Model file for the job. Use its own axes, mm. A direction names the side the tool comes from. Give positions to 0.01 mm unless a question says otherwise; leave off trailing zeros. Loops run counter-clockwise (first coordinate to the right, second up) from the corner with the lowest first, then second, coordinate; pieces in that order, holes last. Notation, with made-up numbers: (68.25, 44.5) - (104.25, 44.5) arc R27 cw to (104.25, 73.5) - close; hole circle Ø1 at (82, 22). An arc over 180 degrees is marked (long way). Use a Markdown table: item, result.
from build123d import *

# Parameters (mm, degrees)
BOSS_EXTRUDE1_DEPTH = 12.7
CUT_EXTRUDE1_DEPTH  = 82.028788994


with BuildPart() as part:
    # Sketch1 → Boss-Extrude1 (new body)
    with BuildSketch(Plane.XY):
        with BuildLine():
            Line((-0.830126662, 34.37418152), (69.93418152, 34.37418152))
            Line((69.93418152, 34.37418152), (69.93418152, -38.90481848))
            Line((69.93418152, -38.90481848), (-41.82581848, -38.90481848))
            Line((-41.82581848, -38.90481848), (-41.82581848, -6.621510298))
            Line((-41.82581848, -6.621510298), (-40.215693332, -5.01138515))
            ThreePointArc((-40.215693332, -5.01138515), (-32.463490161, 0.197163401), (-37.672038711, 7.949366571))
            Line((-37.672038711, 7.949366571), (-41.802956527, 12.080284387))
            Line((-41.802956527, 12.080284387), (-19.531921346, 34.351319567))
            Line((-19.531921346, 34.351319567), (-15.401003531, 30.220401752))
            ThreePointArc((-15.401003531, 30.220401752), (-7.64880036, 25.011853201), (-2.44025181, 32.764056372))
            Line((-2.44025181, 32.764056372), (-0.830126662, 34.37418152))
        make_face()
    extrude(amount=BOSS_EXTRUDE1_DEPTH)

    # Sketch2 → Cut-Extrude1 (cut, through all)
    with BuildSketch(Plane(origin=(0, 0, 0), x_dir=(-1, 0, 0), z_dir=(0, 0, -1))):
        with BuildLine():
            Line((-26.75418152, -4.36081848), (-16.59418152, -4.36081848))
            ThreePointArc((-16.59418152, -4.36081848), (-12.14918152, -8.80581848), (-16.59418152, -13.25081848))
            Line((-16.59418152, -13.25081848), (-26.75418152, -13.25081848))
            ThreePointArc((-26.75418152, -13.25081848), (-31.19918152, -8.80581848), (-26.75418152, -4.36081848))
        make_face()
    extrude(amount=-CUT_EXTRUDE1_DEPTH, mode=Mode.SUBTRACT)


solid = part.part
(1) Slice it at A-A, the plane x = 24. Write the cut outline in (y, z).
Computed:
| item | result |
|---|---|
| outline | (-38.9, 0) - (-13.25, 0) - (-13.25, 12.7) - (-38.9, 12.7) - close; (-4.36, 0) - (34.37, 0) - (34.37, 12.7) - (-4.36, 12.7) - close |
(2) 3-axis set-ups, long thin cutter, end or side, ignore diameter. For faces 4 (the flat face through (15, -38.905, 6)), 5 (the cylindrical face through (31.2, -8.9, 6.3)), 6 (the flat face through (-17.495, 32.315, 6.261)), 7 (the flat face through (-39.71, 9.99, 6.26)): which of +Z, -Z, +X, -X, +Y, -Y reach the whole face in a straight line?
Computed:
| item | result |
|---|---|
| face 4 | +Z, -Z, +X, -X, -Y |
| face 5 | +Z, -Z |
| face 6 | +Z, -Z, +Y |
| face 7 | +Z, -Z, -X |
(3) Pin check, flat tip, straight feed: P1, Ø10, axis at x = 28, y = 4, coming from the -Z side. Stop position of the tip, or through.
Computed:
| item | result |
|---|---|
| P1 | z = 0 |
(4) Slice it at D-D, the plane x = -29. Write the cut outline in (y, z).
Computed:
| item | result |
|---|---|
| outline | (-38.9, 0) - (24.88, 0) - (24.88, 12.7) - (-38.9, 12.7) - close |
(5) Drill centre lines: probe 1 along X at (y, z) = (-8.5, 4.25); probe 2 along X at (y, z) = (-6, 10.25); probe 3 along Y at (x, z) = (-34, 6.25). Where is each one in solid material? Low to high. Write a range as [from, to].
Computed:
| item | result |
|---|---|
| probe 1 | [-41.83, 12.16], [31.19, 69.93] |
| probe 2 | [-41.2, 13.15], [30.2, 69.93] |
| probe 3 | [-38.9, -2.91], [5.85, 19.88] |
(6) Mould opens along X. For faces 1 (the cylindrical face through (12.15, -8.71, 6.26)), 2 (the flat face through (15, -2, 12.7)), 3 (the flat face through (-30.823, 23.06, 6.261)) say: pulls with the +X half, pulls with the -X half, needs draft (parallel to the pull), parting line crosses it, or undercut.
Computed:
| item | result |
|---|---|
| face 1 | undercut |
| face 2 | needs draft |
| face 3 | pulls with the -X half |
(7) Slice it at B-B, the plane y = 26. Write the cut outline in (x, z), plus the area to 3 significant figures.
Computed:
| item | result |
|---|---|
| outline | (-27.88, 0) - (-12.59, 0) - (-12.59, 12.7) - (-27.88, 12.7) - close; (-5.25, 0) - (69.93, 0) - (69.93, 12.7) - (-5.25, 12.7) - close |
| area | 1,150 mm² |
(8) Slice it at C-C, the plane z = 9.25. Write the cut outline in (x, y) (3 decimals).
Computed:
| item | result |
|---|---|
| outline | (-41.826, -38.905) - (69.934, -38.905) - (69.934, 34.374) - (-0.83, 34.374) - (-2.44, 32.764) arc R6.604 cw to (-15.401, 30.22) - (-19.532, 34.351) - (-41.803, 12.08) - (-37.672, 7.949) arc R6.604 cw to (-40.216, -5.011) - (-41.826, -6.622) - close; hole (16.594, -13.251) - (26.754, -13.251) arc R4.445 ccw to (26.754, -4.361) - (16.594, -4.361) arc R4.445 ccw to start |
